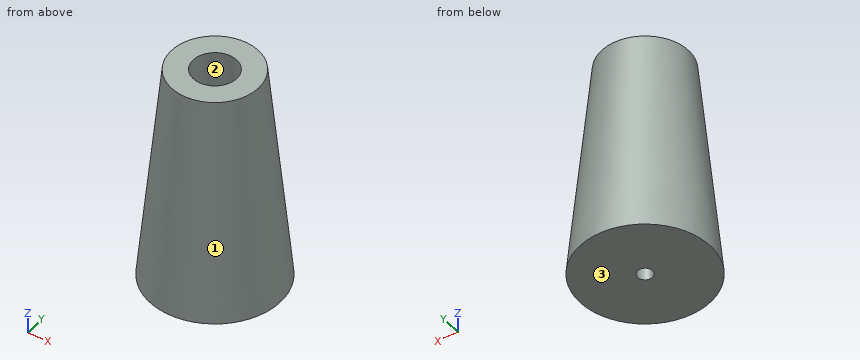
Autodesk Inventor part; units mm, degrees
ref_plane "Work Plane1" through (0, 0, 50) normal (0, 0, 1) x (1, 0, 0)
ref_plane "YZ Plane" through (0, 0, 0) normal (1, 0, 0) x (0, 1, 0)
ref_plane "XZ Plane" through (0, 0, 0) normal (0, 1, 0) x (-1, 0, 0)
sketch "Sketch1" plane through (0, 0, 0) normal (0, 0, 1) x (1, 0, 0)
  circle A0 centre (0, 0) radius 15
  dimension "d0" = 30
ref_plane "Work Plane1" through (0, 0, 50) normal (0, 0, 1) x (1, 0, 0)
sketch "Sketch2" plane through (0, 0, 50) normal (0, 0, 1) x (1, 0, 0)
  circle A0 centre (0, 0) radius 10
  dimension "d2" = 20
loft "Loft1" add profiles "Sketch1", "Sketch2"
sketch "Sketch3" plane through (0, 0, 50) normal (0, 0, 1) x (1, 0, 0)
  circle A0 centre (0, 0) radius 5
  dimension "d7" = 10
extrude "Extrusion1" cut sketch "Sketch3" against normal blind 47
sketch "Sketch4" plane through (0, 0, 0) normal (0, 0, -1) x (-1, 0, 0)
  circle A0 centre (0, 0) radius 1.75
  dimension "d10" = 3.5
extrude "Extrusion2" cut sketch "Sketch4" against normal blind 10
properties part number "training_wheels"
Could you check a few things on this model? Use its own coordinates, in mm. Face numbers are marked on the shaded views. Give positions to 0.01 mm unless a question says otherwise; leave off trailing zeros. Loops run counter-clockwise (first coordinate to the right, second up) from the corner with the lowest first, then second, coordinate; pieces in that order, holes last. Notation, with made-up numbers: (11, 79.5) -> (68, 79.5) arc R16 cw to (68, 93.5) -> close; hole circle Ø3 at (60, 76.5). An arc over 180 degrees is marked (long way). Put each result on its own line as item: value.
(1) I'm going to push flat-ended pins straight in: pin 1 Ø8 at (y, z) = (-0.5, 10) entering from +X; pin 2 Ø4 at (x, z) = (3.5, 37.5) entering from -Y; pin 3 Ø12 at (y, z) = (-4, 21.5) entering from -X. Where does each tip first touch, or does it pass through?
Computed:
pin 1: x = 14.4
pin 2: y = -11.21
pin 3: x = -13.33
(2) Thinking about a two-plate mould opening in X: for the marked faces 1, 2 and 3, which applies, pulls with the +X half, pulls with the -X half, needs draft (parallel to the pull), parting line crosses it, or undercut?
Computed:
face 1: parting line crosses it
face 2: undercut
face 3: needs draft
(3) Imagine slicing it at A-A on x = 0. Write out the boundary of the cut face in (y, z), plus the area to 4 significant figures.
Computed:
outline: (-15, 0) -> (-1.75, 0) -> (-1.75, 3) -> (-5, 3) -> (-5, 50) -> (-10, 50) -> close; (1.75, 0) -> (15, 0) -> (10, 50) -> (5, 50) -> (5, 3) -> (1.75, 3) -> close
area: 769.5 mm^2
(4) Imagine slicing it at C-C on z = 45.5. Write out the boundary of the cut face in (x, y), plus the area to 3 significant figures.
Computed:
outline: circle Ø20.9 at (0, 0); hole circle Ø10 at (0, 0)
area: 265 mm^2
(5) Please list where these lines run through material, in increasing order: probe 1 along Z at (x, y) = (0.5, -4); probe 2 along Y at (x, z) = (-2, 41); probe 3 along Y at (x, z) = (0, 14). Write a range as [from, to].
Computed:
probe 1: [0, 3]
probe 2: [-10.71, -4.58], [4.58, 10.71]
probe 3: [-13.6, -5], [5, 13.6]
(6) Imagine slicing it at B-B on z = 33. Write out the boundary of the cut face in (x, y).
Computed:
outline: circle Ø23.4 at (0, 0); hole circle Ø10 at (0, 0)
